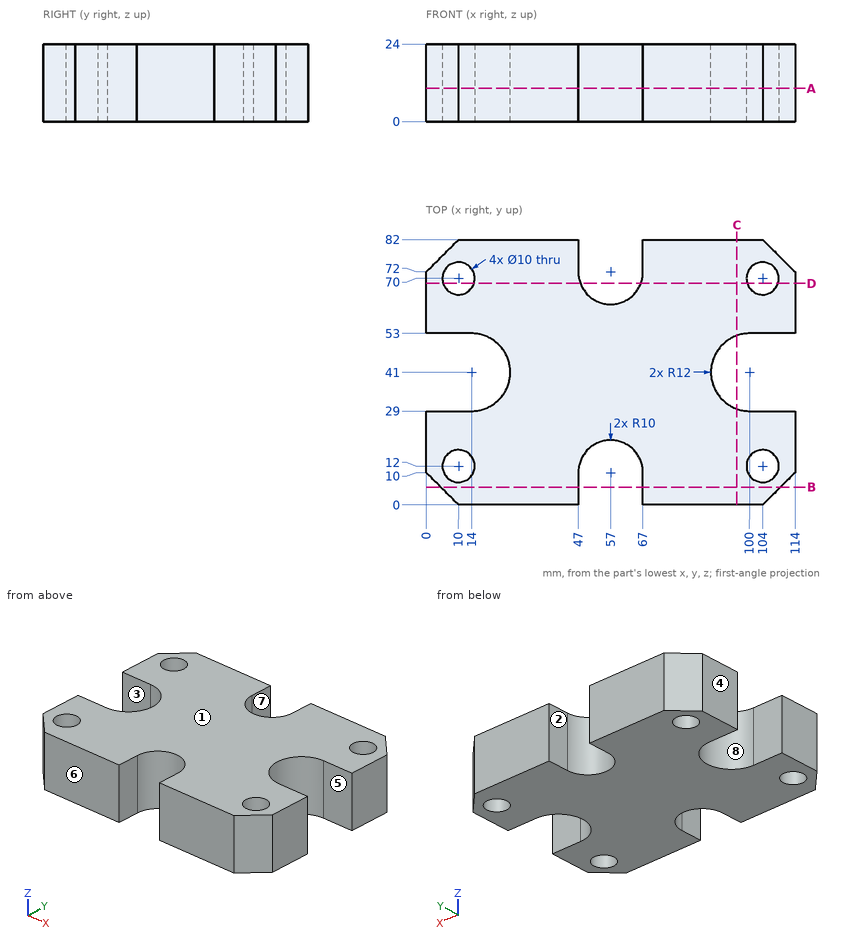
Answer from the drawing. Dimensions are ordinates in mm from the lowest x, y and z of the part. A direction names the side the tool comes from. Coordinates: 2 decimals unless noted, no trailing zeros. Write each loop counter-clockwise with the first axis right and the second up, starting at its lowest first coordinate (ties: lowest second). Pieces come first, ordered by that corner, then holes. Notation, with made-up numbers: M -14.5,40 L 0.5,40 A15 cw 0.5,56 Z; hole C 69.25,24 d6. An arc over 180 degrees is marked long. Put each result on its own line as item: value. Start each with the question number.
1. Flat-ended cylindrical pins translate along their axes: P1, Ø8, axis at y = 4.5, z = 16.5, coming from the +X side; P2, Ø3, axis at x = 71.5, z = 20, coming from the -Y side; P3, Ø8, axis at x = 104, y = 70, coming from the -Z side; P4, Ø7, axis at x = 4.5, z = 10, coming from the +Y side. Find the tip coordinate at first contact, or state that the pin passes through.
2. Consider line 1 (Y direction, x = 10, z = 7.5); line 2 (X direction, y = 8, z = 13.5); line 3 (Y direction, x = 13, z = 17). Determine where each line is inside the solid, lowest interval first. Write a range as from..to.
3. Which of the six approach directions +Z, -Z, +X, -X, +Y, -Y give full straight-line access (tool end or side, diameter ignored) to the marked faces 1, 2, 3, 4 and 5?
4. For a pull along Y with two mould halves and no side action, classify the marked faces 6, 7 and 8 as pulls with the +Y half, pulls with the -Y half, needs draft (parallel to the pull), parting line crosses it, or undercut.
5. A cutting plane is placed at A-A on z = 10.25. Write down the section's boundary in (x, y).
6. A cutting plane is placed at D-D on y = 68.5. Write down the section's boundary in (x, z).
7. A cutting plane is placed at B-B on y = 5.5. Write down the section's boundary in (x, z), then the cut area to 3 significant figures.
8. A cutting plane is placed at C-C on x = 96. Write down the section's boundary in (y, z), then the cut area to 3 significant figures.
Resolved:
1. P1: stops at x = 112.5
1. P2: stops at y = 0
1. P3: passes through
1. P4: stops at y = 80
2. line 1: y = 0..7, 17..29, 53..65, 75..82
2. line 2: x = 2..7, 13..47, 67..101, 107..112
2. line 3: y = 0..8, 16..29, 53..66, 74..82
3. face 1: +Z, +X, -X, +Y, -Y
3. face 2: +Z, -Z, +Y
3. face 3: +Z, -Z, -X
3. face 4: +Z, -Z, -X, +Y, -Y
3. face 5: +Z, -Z, +X
4. face 6: pulls with the -Y half
4. face 7: needs draft
4. face 8: undercut
5. outline: M 0,10 L 10,0 L 47,0 L 47,10 A10 cw 67,10 L 67,0 L 104,0 L 114,10 L 114,29 L 100,29 A12 cw 100,53 L 114,53 L 114,72 L 104,82 L 67,82 L 67,72 A10 cw 47,72 L 47,82 L 10,82 L 0,72 L 0,53 L 14,53 A12 cw 14,29 L 0,29 Z; hole C 10,12 d10; hole C 10,70 d10; hole C 104,12 d10; hole C 104,70 d10
6. outline: M 0,0 L 5.23,0 L 5.23,24 L 0,24 Z; M 14.77,0 L 47.63,0 L 47.63,24 L 14.77,24 Z; M 66.37,0 L 99.23,0 L 99.23,24 L 66.37,24 Z; M 108.77,0 L 114,0 L 114,24 L 108.77,24 Z
7. outline: M 4.5,0 L 47,0 L 47,24 L 4.5,24 Z; M 67,0 L 109.5,0 L 109.5,24 L 67,24 Z
7. area: 2,040 mm2
8. outline: M 0,0 L 29.69,0 L 29.69,24 L 0,24 Z; M 52.31,0 L 82,0 L 82,24 L 52.31,24 Z
8. area: 1,420 mm2
